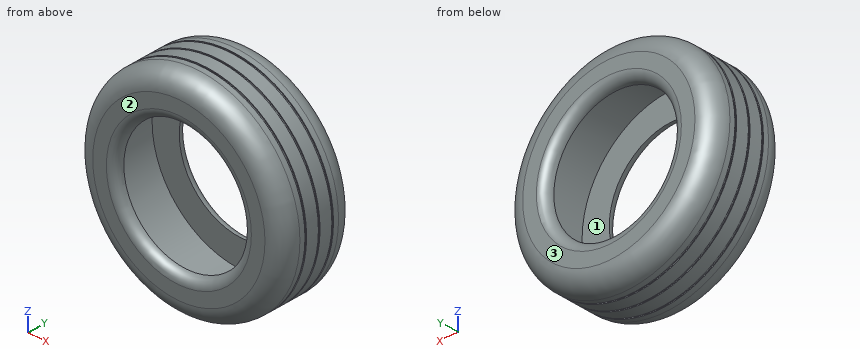
from build123d import *

# Parameters (mm, degrees)
F0_R     = 575
F1_DEPTH = 430
F2_R     = 350
F3_DEPTH = 500
F4_R     = 100
F5_R     = 50
F6_W     = 148.077123
F6_H     = 10
F6_W_2   = 157.069139
F6_W_3   = 114.678197


with BuildPart() as f1:
    # F0 (on Front) → F1 (new body)
    with BuildSketch(Plane.XZ):
        Circle(F0_R)
    extrude(amount=F1_DEPTH)

    # F2 (on face) → F3 (cut)
    with BuildSketch(Plane.XZ.offset(430)):
        Circle(F2_R)
    extrude(amount=-F3_DEPTH, mode=Mode.SUBTRACT)

    # F4
    f4_edges = [f1.edges().sort_by_distance(p)[0] for p in [
        (-575, -430, 0),
        (-575, 0, 0),
    ]]
    fillet(f4_edges, radius=F4_R)

    # F5
    f5_edges = [f1.edges().sort_by_distance(p)[0] for p in [
        (-350, -430, 0),
        (-350, 0, 0),
    ]]
    fillet(f5_edges, radius=F5_R)

    # F6 (on Top) → F7 (revolve, cut)
    with BuildSketch(Plane.XY):
        Polygon((350, 0), (0, 0), (0, -430), (350, -430), (350, -380), (500, -380), (500, -50), (350, -50), align=None)
        with Locations((644.038562, -295)):
            Rectangle(F6_W, F6_H)
        with Locations((648.534569, -215)):
            Rectangle(F6_W_2, F6_H)
        with Locations((627.339098, -135)):
            Rectangle(F6_W_3, F6_H)
    revolve(axis=Axis((0, -215, 0), (0, 1, 0)), mode=Mode.SUBTRACT)


solid = f1.part
The model under review builds one solid part; all positions refer to its coordinate system, in mm. Face numbers are marked on the shaded views. Coordinates: 2 decimals unless noted, no trailing zeros. Loops run counter-clockwise (first coordinate to the right, second up) from the corner with the lowest first, then second, coordinate; pieces in that order, holes last. Notation, with made-up numbers: (74.5, -27) -> (110.5, -27) arc R26 cw to (110.5, 9) -> close; hole circle Ø5 at (-17.5, 37.5). An arc over 180 degrees is marked (long way). Use a Markdown table: item, result. Add a question column.
1. Draft analysis for pull direction Y (two halves, no side actions). For the marked faces 1, 2 and 3, state which applies: pulls with the +Y half, pulls with the -Y half, needs draft (parallel to the pull), parting line crosses it, or undercut.
2. Clearance check with flat-ended pins moving along their axes: pin 1 Ø12 at (x, z) = (245, 442.5) entering from +Y; pin 2 Ø2 at (y, z) = (-185.5, -142.5) entering from +X; pin 3 Ø12 at (x, y) = (270.5, -129.5) entering from -Z. State where each tip first meets the part, or that it passes through.
3. Add section A-A on y = -67.5. Write out the cut boundary in (x, z), plus the area to 3 significant figures.
4. To check wall thickness, follow line 1 (X direction, y = -234, z = 0); line 2 (Y direction, x = -306.5, z = -306.5); line 3 (Z direction, x = 0, y = -219). State the ranges of each line that lie inside material, in increasing order.
Returned:
| question | item | result |
|---|---|---|
| 1 | face 1 | undercut |
| 1 | face 2 | pulls with the -Y half |
| 1 | face 3 | pulls with the +Y half |
| 2 | pin 1 | stops at y = -3.12 |
| 2 | pin 2 | stops at x = 557.32 |
| 2 | pin 3 | stops at z = -510.55 |
| 3 | outline | circle Ø1139.14 at (0, 0); hole circle Ø1000 at (0, 0) |
| 3 | area | 234,000 mm² |
| 4 | line 1 | x = -575 to -500, 500 to 575 |
| 4 | line 2 | y = -430 to -380, -50 to 0 |
| 4 | line 3 | z = -570 to -500, 500 to 570 |
